The model under review builds one solid part; all positions refer to its coordinate system, in mm. A direction names the side the tool comes from. Round coordinates to 2 decimals unless told otherwise and drop trailing zeros. Order: outer loops, then holes, each group sorted by start corner. A loop starts at its lowest first (then second) coordinate and runs counter-clockwise, first axis right, second up. Notation, with made-up numbers: M 44,89.25 L 72,89.25 A16 cw 72,115.25 Z; hole C 37.5,-4 d7. An arc over 180 degrees is marked long. Answer as a JSON object with one key per item and string values. Group by question number.
1. To check wall thickness, follow probe 1 along X at (y, z) = (-3, -41.5); probe 2 along Z at (x, y) = (-31, -3); probe 3 along Z at (x, y) = (-18, -3.5). State the ranges of each line that lie inside material, in increasing order. Write a range as [from, to].
2. Mouldability with a two-part tool opening along X and no side actions: class faces 1 (the face through (-67.125, -3, 8)), 2 (the face through (-34, 0, 8)), 3 (the face through (-3.264, -4.729, -58.626)) as released by +X, released by -X, zero draft, split by the parting line, or undercut.
3. Machinability: for faces 4 (the face through (-34, -3, -61.93)), 5 (the face through (-64.585, -5, 8)), which of the approach directions +Z, -Z, +X, -X, +Y, -Y give a long, thin tool a straight path to every point of the face, cutting with its end or side? Answer none if there is none.
4. Add section D-D on z = 67. State the section outline as (x, y) points, and give its area (3 significant figures).
5. Add section A-A on y = -5.5. State the section outline as (x, z) points.
6. Add section B-B on z = 20. State the section outline as (x, y) points.
7. Clearance check with flat-ended pins moving along their axes: P1, Ø4, axis at x = -22.5, z = 15, coming from the -Y side; P2, Ø3, axis at x = -60.5, z = -35, coming from the +Y side; P3, Ø2, axis at x = -36.5, y = -4.5, coming from the +Z side. State where each tip first meets the part, or that it passes through.
8. Add section C-C on x = -17.5. State the section outline as (y, z) points.
```python
from build123d import *

# Parameters (mm, degrees)
F1_DEPTH = 6.858
F2_R     = 5.08
F3_R     = 6.181057
F4_DEPTH = 6.858
F6_T     = -2.54


with BuildPart() as f1:
    # F0 (on Front) → F1 (new body)
    with BuildSketch(Plane.XZ):
        Polygon((0, -61.929818), (0, 76.246182), (-67.125276, 76.269276), (-67.125276, -61.929818), align=None)
    extrude(amount=F1_DEPTH)

    # F2
    f2_edges = [f1.edges().sort_by_distance(p)[0] for p in [
        (-67.125276, -3.429, 76.269276),
        (0, -3.429, -61.929818),
        (-67.125276, -3.429, -61.929818),
        (0, -3.429, 76.246182),
    ]]
    fillet(f2_edges, radius=F2_R)

    # F3 (on face) → F4 (cut)
    with BuildSketch(Plane.XZ.offset(6.858)):
        with Locations((-13.514167, 63.706279)):
            Circle(F3_R)
    extrude(amount=-F4_DEPTH, mode=Mode.SUBTRACT)

    # F6
    f6_openings = [f1.faces().sort_by_distance(p)[0] for p in [
        (-33.827013, -6.858, 6.420933),
    ]]
    offset(amount=F6_T, openings=f6_openings)


solid = f1.part
```
Recorded:
{
 "1": {"probe 1": "x = [-67.13, -64.59], [-2.54, 0]", "probe 2": "z = [-61.93, -59.39], [73.72, 76.26]", "probe 3": "z = [-61.93, -59.39], [56.23, 59.45], [67.96, 71.19], [73.71, 76.25]"},
 "2": {"face 1": "released by -X", "face 2": "zero draft", "face 3": "undercut"},
 "3": {"face 4": "-Z, +X, -X, +Y, -Y", "face 5": "-Y"},
 "4": {"outline": "M -67.13,-6.86 L -64.59,-6.86 L -64.59,-2.54 L -21.59,-2.54 L -21.59,-6.86 L -18.74,-6.86 L -18.74,0 L -67.13,0 Z; M -8.28,-6.86 L -5.44,-6.86 L -5.44,-2.54 L -2.54,-2.54 L -2.54,-6.86 L 0,-6.86 L 0,0 L -8.28,0 Z", "area": "190 mm²"},
 "5": {"outline": "M -67.13,-56.85 A5.08 ccw -62.05,-61.93 L -5.08,-61.93 A5.08 ccw 0,-56.85 L 0,71.17 A5.08 ccw -5.08,76.25 L -62.04,76.27 A5.08 ccw -67.13,71.19 Z; C -13.51,63.71 d17.44; hole M -64.59,-56.85 A2.54 ccw -62.05,-59.39 L -5.08,-59.39 A2.54 ccw -2.54,-56.85 L -2.54,71.17 A2.54 ccw -5.08,73.71 L -62.04,73.73 A2.54 ccw -64.59,71.19 Z; hole C -13.51,63.71 d12.36"},
 "6": {"outline": "M -67.13,-6.86 L -64.59,-6.86 L -64.59,-2.54 L -2.54,-2.54 L -2.54,-6.86 L 0,-6.86 L 0,0 L -67.13,0 Z"},
 "7": {"P1": "stops at y = -2.54", "P2": "stops at y = 0", "P3": "stops at z = 76.26"},
 "8": {"outline": "M -6.86,-61.93 L 0,-61.93 L 0,58.98 L -6.86,58.98 L -6.86,55.95 L -2.54,55.95 L -2.54,-59.39 L -6.86,-59.39 Z; M -6.86,68.43 L 0,68.43 L 0,76.25 L -6.86,76.25 L -6.86,73.71 L -2.54,73.71 L -2.54,71.46 L -6.86,71.46 Z"}
}
